Read the model definition and answer for the solid it produces. Units are mm, in the model's axes. A direction names the side the tool comes from. Give positions to 0.01 mm unless a question says otherwise; leave off trailing zeros. Write each loop counter-clockwise with the first axis right and the second up, starting at its lowest first coordinate (ties: lowest second). Pieces come first, ordered by that corner, then holes. Notation, with made-up numbers: M 42.25,26 L 81.25,26 A16 cw 81.25,36 Z; hole C 71.5,-37.75 d7. An arc over 180 degrees is marked long. Use a Markdown table: item, result. Add a question column.
Item 1: The mould has two halves that part along Z. Classify faces 1 (the flat face through (1, 0, 61)), 2 (the flat face through (26, 2, 70)), 3 (the cylindrical face through (28.575, 1.972, -64.186)), 4 (the flat face through (-70, 2, 1)): pulls with the +Z half, pulls with the -Z half, needs draft (parallel to the pull), parting line crosses it, or undercut.
Item 2: A cutting plane is placed at B-B on z = 31.5. Determine the outline of the cut face in (x, y), then the cut area to 3 significant figures.
Item 3: A cutting plane is placed at A-A on y = 1.6. Count the separate pieces of the cut face and the enclosed holes in it, then the cut area to 3 significant figures.
Item 4: A cutting plane is placed at C-C on x = -53. Determine the outline of the cut face in (y, z), then the cut area to 3 significant figures.
Item 5: For faces 5 (the flat face through (26, 2, 55)), 6 (the flat face through (-85, 2, 1)), determine the directions among +Z, -Z, +X, -X, +Y, -Y from which every point of the face is accessible in a straight line to the end or side of a thin tool.
Item 6: Consider probe 1 along Z at (x, y) = (132.5, 2.9); probe 2 along X at (y, z) = (2, 62.5); probe 3 along X at (y, z) = (1.5, 0). Determine where each line is inside the solid, lowest interval first. Write a range as [from, to].
from build123d import *

# Parameters (mm, degrees)
SKETCH1_W           = 225
SKETCH1_H           = 140
SKETCH1_R           = 2
SKETCH1_W_2         = 195
SKETCH1_H_2         = 110
BOSS_EXTRUDE1_DEPTH = 4


with BuildPart() as part:
    # Sketch1 → Boss-Extrude1 (new body)
    with BuildSketch(Plane(origin=(0, 0, 0), x_dir=(1, 0, 0), z_dir=(0, 1, 0))):
        with Locations((27.5, 0)):
            Rectangle(SKETCH1_W, SKETCH1_H)
        with Locations((-77.5, -62.5)):
            Circle(SKETCH1_R, mode=Mode.SUBTRACT)
        with Locations((-77.5, 62.5)):
            Circle(SKETCH1_R, mode=Mode.SUBTRACT)
        with Locations((132.5, 62.5)):
            Circle(SKETCH1_R, mode=Mode.SUBTRACT)
        with Locations((132.5, -62.5)):
            Circle(SKETCH1_R, mode=Mode.SUBTRACT)
        with Locations((27.5, -62.5)):
            Circle(SKETCH1_R, mode=Mode.SUBTRACT)
        with Locations((27.5, 62.5)):
            Circle(SKETCH1_R, mode=Mode.SUBTRACT)
        with Locations((-77.5, 0)):
            Circle(SKETCH1_R, mode=Mode.SUBTRACT)
        with Locations((132.5, 0)):
            Circle(SKETCH1_R, mode=Mode.SUBTRACT)
        with Locations((27.5, 0)):
            Rectangle(SKETCH1_W_2, SKETCH1_H_2, mode=Mode.SUBTRACT)
    extrude(amount=BOSS_EXTRUDE1_DEPTH)


solid = part.part
Filled in:
| question | item | result |
|---|---|---|
| 1 | face 1 | needs draft |
| 1 | face 2 | pulls with the +Z half |
| 1 | face 3 | undercut |
| 1 | face 4 | undercut |
| 2 | outline | M -85,0 L -70,0 L -70,4 L -85,4 Z; M 125,0 L 140,0 L 140,4 L 125,4 Z |
| 2 | area | 120 mm² |
| 3 | separate pieces | 1 |
| 3 | enclosed holes | 9 |
| 3 | area | 9,950 mm² |
| 4 | outline | M 0,-70 L 4,-70 L 4,-55 L 0,-55 Z; M 0,55 L 4,55 L 4,70 L 0,70 Z |
| 4 | area | 120 mm² |
| 5 | face 5 | +Y, -Y |
| 5 | face 6 | +Z, -Z, -X, +Y, -Y |
| 6 | probe 1 | [-70, -64.5], [-60.5, -2], [2, 60.5], [64.5, 70] |
| 6 | probe 2 | [-85, -79.5], [-75.5, 25.5], [29.5, 130.5], [134.5, 140] |
| 6 | probe 3 | [-85, -79.5], [-75.5, -70], [125, 130.5], [134.5, 140] |
